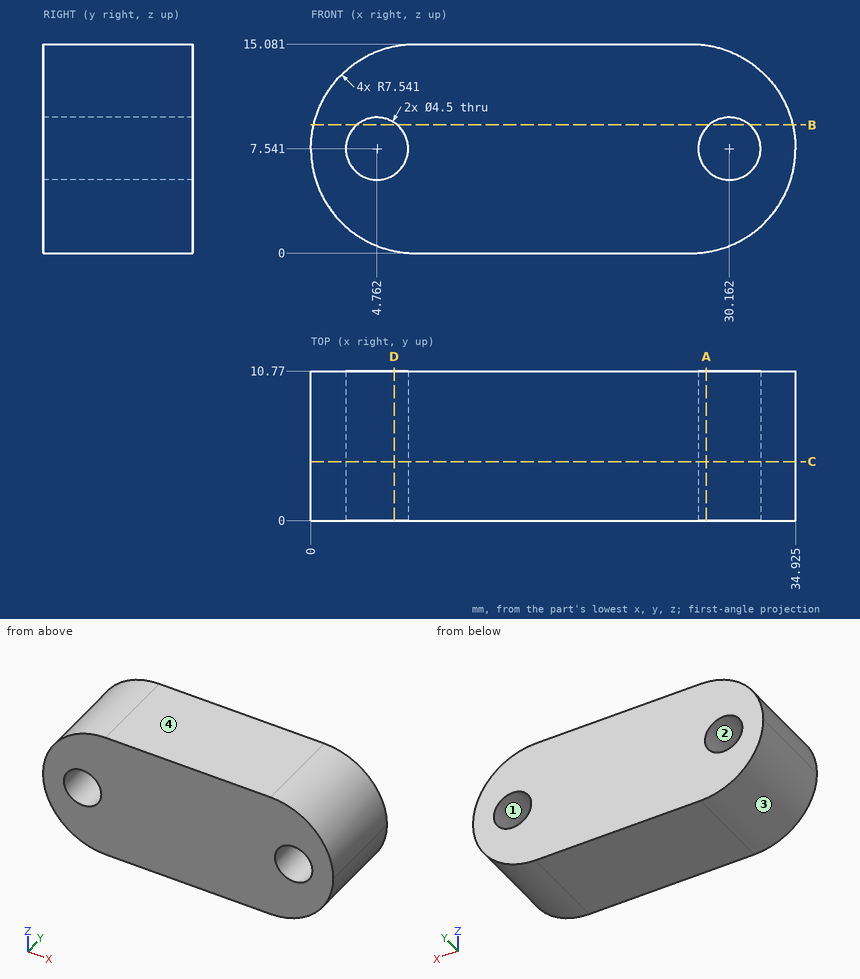
The drawing under review shows one solid part. Ordinate dimensions are in mm from its lowest x, y, z. Coordinates: 2 decimals unless noted, no trailing zeros. Order: outer loops, then holes, each group sorted by start corner. A loop starts at its lowest first (then second) coordinate and runs counter-clockwise, first axis right, second up. Notation, with made-up numbers: (-22, -28.5) - (-17, -28.5) arc R16 cw to (-17, -3.5) - close; hole circle Ø7 at (-25, 35.25). An arc over 180 degrees is marked (long way). Put each result on its own line as item: value.
1) The part is to be moulded in two halves that separate along Z. For the marked faces 1, 2, 3 and 4, say which applies: released by +Z, released by -Z, zero draft, split by the parting line, or undercut.
Response values:
face 1: undercut
face 2: undercut
face 3: released by -Z
face 4: released by +Z
2) Insertion check: P1, Ø6, axis at y = 4, z = 11, coming from the +X side; P2, Ø2, axis at y = 4.5, z = 10.5, coming from the +X side; P3, Ø4, axis at y = 8, z = 13, coming from the -X side. Each pin has a flat end and moves straight along its axis. Give the tip position at first contact, or say it passes through.
Response values:
P1: stops at x = 34.91
P2: stops at x = 34.67
P3: stops at x = 0.84
3) Take a section at B-B, the plane z = 9.25. Give the boundary of the cut face in (x, y) (1 decimal).
Response values:
outline: (0.2, 0) - (3.3, 0) - (3.3, 10.8) - (0.2, 10.8) - close; (6.2, 0) - (28.7, 0) - (28.7, 10.8) - (6.2, 10.8) - close; (31.6, 0) - (34.7, 0) - (34.7, 10.8) - (31.6, 10.8) - close
4) Take a section at C-C, the plane y = 4.25. Count the separate pieces of the cut face and the enclosed holes in it, and give its area (3 significant figures).
Response values:
separate pieces: 1
enclosed holes: 2
area: 446 mm²
5) Take a section at D-D, the plane x = 6. Give the boundary of the cut face in (y, z).
Response values:
outline: (0, 0.16) - (10.77, 0.16) - (10.77, 5.66) - (0, 5.66) - close; (0, 9.42) - (10.77, 9.42) - (10.77, 14.92) - (0, 14.92) - close
6) Wall thickness on L1, parallel to X at y = 7.5, z = 5.5 (1 decimal); L2, parallel to X at y = 8.5, z = 7 (1 decimal); L3, parallel to Z at x = 3.5, y = 9 (1 decimal): over which ranges is each line inside the solid? List them lowest first. Write a range as from..to.
Response values:
L1: x = 0.3..3.8, 5.7..29.2, 31.1..34.6
L2: x = 0..2.6, 6.9..28, 32.3..34.9
L3: z = 1.2..5.7, 9.4..13.9
7) Take a section at A-A, the plane x = 28.5. Give the boundary of the cut face in (y, z) (1 decimal).
Response values:
outline: (0, 0.1) - (10.8, 0.1) - (10.8, 6) - (0, 6) - close; (0, 9.1) - (10.8, 9.1) - (10.8, 15) - (0, 15) - close
